Autodesk Inventor part; units mm, degrees
ref_plane "Work Plane1" through (0, -138.176, 0) normal (1, 0, 0) x (0, 1, 0)
ref_plane "YZ Plane" through (0, 0, 0) normal (1, 0, 0) x (0, 1, 0)
ref_plane "XZ Plane" through (0, 0, 0) normal (0, 1, 0) x (-1, 0, 0)
sketch "Sketch1" plane through (0, 0, 0) normal (0, 0, 1) x (1, 0, 0)
  line L0 (-295.275, -138.176) -> (295.275, -138.176)
  line L1 (295.275, -138.176) -> (295.275, 138.176)
  line L2 (295.275, 138.176) -> (-295.275, 138.176)
  line L3 (-295.275, 138.176) -> (-295.275, -138.176)
  line L4 (-295.275, -138.176) -> (295.275, 138.176) construction
  line L5 (295.275, -138.176) -> (-295.275, 138.176) construction
  point P0 (0, 0)
  dimension "d0" = 590.55
  dimension "d1" = 276.352
extrude "Extrusion1" add sketch "Sketch1" against normal blind 6.35
sketch "Sketch2" plane through (0, 0, 0) normal (0, 0, 1) x (1, 0, 0)
  line L0 (-295.275, -138.176) -> (295.275, -138.176)
  line L1 (295.275, 138.176) -> (-295.275, 138.176)
  line L2 (-295.275, 138.176) -> (-295.275, -138.176)
  line L3 (-295.275, 93.726) -> (-250.825, 93.726)
  line L4 (-250.825, 93.726) -> (-250.825, 138.176)
  point P0 (0, 0)
  dimension "d4" = 44.45
  dimension "d6" = 231.902
extrude "Extrusion2" cut sketch "Sketch2" against normal through all
fillet "Fillet1" radius 6.35 1 edges at (-250.825, 93.726, -3.175)
ref_plane "Work Plane1" through (0, -138.176, 0) normal (1, 0, 0) x (0, 1, 0)
mirror "Mirror1" about plane through (0, -138.176, 0) normal (1, 0, 0) of "Extrusion2", "Fillet1"
sketch "Sketch3" plane through (0, 0, 0) normal (0, 0, 1) x (1, 0, 0)
  line L0 (-295.275, 93.726) -> (-295.275, -138.176)
  line L1 (-295.275, -138.176) -> (295.275, -138.176)
  point P0 (0, 0)
  point P1 (-228.473, -122.174)
  point P2 (244.475, -122.174)
  dimension "d10" = 66.802
  dimension "d11" = 539.75
  dimension "d12" = 16.002
hole "Hole1" at (-228.473, -122.174, 0) at (244.475, -122.174, 0) direction (0, 0, -1) diameter 6.858 end through all
properties part number "GE-13042" material "Polycarbonate, Clear"
Model file for the job. Use its own axes, mm. Coordinates: 2 decimals unless noted, no trailing zeros. Write each loop counter-clockwise with the first axis right and the second up, starting at its lowest first coordinate (ties: lowest second). Pieces come first, ordered by that corner, then holes. Notation, with made-up numbers: (43, 86.25) - (63, 86.25) arc R23 cw to (63, 125.25) - close; hole circle Ø4 at (39, 41.5). An arc over 180 degrees is marked (long way). Use a Markdown table: item, result. Add a question column.
Item 1: Drop flat-ended pins along their axis: pin 1 (1.9 mm diameter, centred on x = 275.5, z = -2.5, fed in from +Y); pin 2 (1.9 mm diameter, centred on y = 125.5, z = -4.5, fed in from +X) (3 decimals); pin 3 (1.9 mm diameter, centred on y = 123.5, z = -4, fed in from -X) (3 decimals). Give the stop position or say it passes through.
Item 2: Drill centre lines: line 1 along Y through (x, z) = (269.5, -0.25); line 2 along X through (y, z) = (109, -5) (3 decimals); line 3 along Y through (x, z) = (-253, -3.75). Where is each one in solid material? Low to high.
Item 3: Band-saw the part on A-A, the plane z = -5.25. Write the cut outline in (x, y) (3 decimals).
A:
| question | item | result |
|---|---|---|
| 1 | pin 1 | stops at y = 93.73 |
| 1 | pin 2 | stops at x = 250.825 |
| 1 | pin 3 | stops at x = -250.825 |
| 2 | line 1 | y = -138.18 to 93.73 |
| 2 | line 2 | x = -250.825 to 250.825 |
| 2 | line 3 | y = -138.18 to 95.29 |
| 3 | outline | (-295.275, -138.176) - (295.275, -138.176) - (295.275, 93.726) - (257.175, 93.726) arc R6.35 cw to (250.825, 100.076) - (250.825, 138.176) - (-250.825, 138.176) - (-250.825, 100.076) arc R6.35 cw to (-257.175, 93.726) - (-295.275, 93.726) - close; hole circle Ø6.858 at (-228.473, -122.174); hole circle Ø6.858 at (244.475, -122.174) |
